```python
from build123d import *

# Parameters (mm, degrees)
F0_R     = 6.5
F0_R_2   = 3
F1_DEPTH = 5
F2_W     = 1.5
F2_H     = 0.5
F5_R     = 0.1
F6_R     = 0.1


with BuildPart() as f1:
    # F0 (on Front) → F1 (new body)
    with BuildSketch(Plane.XZ):
        Circle(F0_R)
        Circle(F0_R_2, mode=Mode.SUBTRACT)
    extrude(amount=F1_DEPTH)

    # F2 (on Top) → F3 (revolve, cut)
    with BuildSketch(Plane.XY):
        with Locations((-4.25, -4.791322)):
            Rectangle(F2_W, F2_H)
    revolve(axis=Axis((0, -1.116181, 0), (0, -1, 0)), mode=Mode.SUBTRACT)

    # F2 (on Top) → F4 (revolve, cut)
    with BuildSketch(Plane.XY):
        with Locations((-4.25, -0.25)):
            Rectangle(F2_W, F2_H)
    revolve(axis=Axis((0, -1.116181, 0), (0, -1, 0)), mode=Mode.SUBTRACT)

    # F5
    f5_edges = [f1.edges().sort_by_distance(p)[0] for p in [
        (-6.5, -5, 0),
    ]]
    fillet(f5_edges, radius=F5_R)

    # F6
    f6_edges = [f1.edges().sort_by_distance(p)[0] for p in [
        (-6.5, 0, 0),
    ]]
    fillet(f6_edges, radius=F6_R)


solid = f1.part
```
Read the model definition and answer for the solid it produces. Units are mm, in the model's axes. A direction names the side the tool comes from. Give positions to 0.01 mm unless a question says otherwise; leave off trailing zeros. Order: outer loops, then holes, each group sorted by start corner. A loop starts at its lowest first (then second) coordinate and runs counter-clockwise, first axis right, second up. Notation, with made-up numbers: (6, -17.5) -> (44, -17.5) arc R28 ccw to (44, 4.5) -> close; hole circle Ø5 at (-20, 59). An arc over 180 degrees is marked (long way). One line per item, written item: value. Start each with the question number.
(1) The part is cut by section C-C (y = -2). Determine the outline of the cut face in (x, z), and give its area (3 significant figures).
(2) Flat-ended cylindrical pins translate along their axes: P1, Ø2, axis at y = -3.5, z = 2, coming from the +X side; P2, Ø1.5, axis at y = -4, z = 1, coming from the +X side; P3, Ø1.5, axis at x = -4, y = -3.5, coming from the -Z side. Find the tip coordinate at first contact, or state that the pin passes through.
(3) The part is cut by section B-B (x = 0). Determine the outline of the cut face in (y, z).
(4) For a pull along X with two mould halves and no side action, classify faces 4 (the cylindrical face through (-5.158, -2.466, -3.955)), 5 (the flat face through (-5, 0, -2)), 6 (the cylindrical face through (-3.233, -0.246, 1.341)) as released by +X, released by -X, zero draft, split by the parting line, or undercut.
(5) The part is cut by section A-A (z = 0). Determine the outline of the cut face in (x, y), and give its area (3 significant figures).
(6) Straight lines are drawn through the part: L1, parallel to Z at x = 0, y = -0.2; L2, parallel to Z at x = 0, y = -1.9; L3, parallel to Z at x = -2.5, y = -0.3. For each, find the intervals that lie inside material, in ascending order.
(7) A tool of negligible diameter and unlimited length cuts with its end or side. For faces 1 (the flat face through (-2.2, -0.5, 3.3)), 2 (the flat face through (-2.2, -4.541, 3.3)), 3 (the flat face through (-5, -5, -2)), from which of +Z, -Z, +X, -X, +Y, -Y can it reach the whole face along a straight path? Write none if from no direction.
Taken from the geometry:
1. outline: circle Ø13 at (0, 0); hole circle Ø6 at (0, 0)
1. area: 104 mm^2
2. P1: x = 6.42
2. P2: x = 6.5
2. P3: z = -5.63
3. outline: (-5, -6.4) arc R0.1 ccw to (-4.9, -6.5) -> (-0.1, -6.5) arc R0.1 ccw to (0, -6.4) -> (0, -5) -> (-0.5, -5) -> (-0.5, -3.5) -> (0, -3.5) -> (0, -3) -> (-5, -3) -> (-5, -3.5) -> (-4.54, -3.5) -> (-4.54, -5) -> (-5, -5) -> close; (-5, 3) -> (0, 3) -> (0, 3.5) -> (-0.5, 3.5) -> (-0.5, 5) -> (0, 5) -> (0, 6.4) arc R0.1 ccw to (-0.1, 6.5) -> (-4.9, 6.5) arc R0.1 ccw to (-5, 6.4) -> (-5, 5) -> (-4.54, 5) -> (-4.54, 3.5) -> (-5, 3.5) -> close
4. face 4: split by the parting line
4. face 5: zero draft
4. face 6: undercut
5. outline: (-6.5, -4.9) arc R0.1 ccw to (-6.4, -5) -> (-5, -5) -> (-5, -4.54) -> (-3.5, -4.54) -> (-3.5, -5) -> (-3, -5) -> (-3, 0) -> (-3.5, 0) -> (-3.5, -0.5) -> (-5, -0.5) -> (-5, 0) -> (-6.4, 0) arc R0.1 ccw to (-6.5, -0.1) -> close; (3, -5) -> (3.5, -5) -> (3.5, -4.54) -> (5, -4.54) -> (5, -5) -> (6.4, -5) arc R0.1 ccw to (6.5, -4.9) -> (6.5, -0.1) arc R0.1 ccw to (6.4, 0) -> (5, 0) -> (5, -0.5) -> (3.5, -0.5) -> (3.5, 0) -> (3, 0) -> close
5. area: 32.1 mm^2
6. L1: -6.5 to -5, -3.5 to -3, 3 to 3.5, 5 to 6.5
6. L2: -6.5 to -3, 3 to 6.5
6. L3: -6 to -4.33, -2.45 to -1.66, 1.66 to 2.45, 4.33 to 6
7. face 1: +Y
7. face 2: -Y
7. face 3: +Z, -Z, +X, -X, -Y
